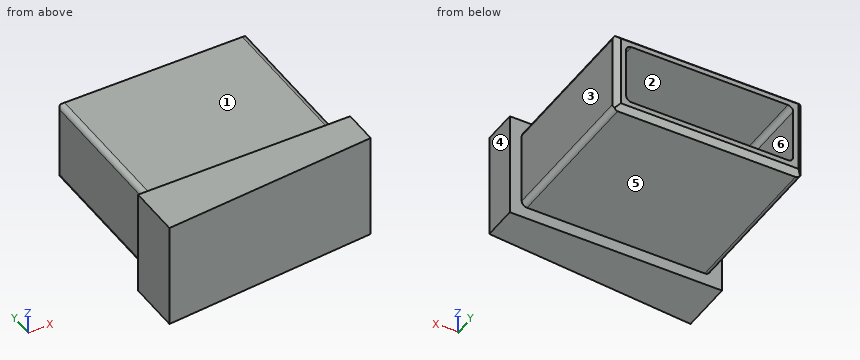
from build123d import *

# Parameters (mm, degrees)
SKETCH1_W           = 45.085
SKETCH1_H           = 38.1
BOSS_EXTRUDE1_DEPTH = 9.8425
SKETCH2_W           = 50.8
SKETCH2_H           = 25.4
BOSS_EXTRUDE2_DEPTH = 12.7635
CUT_EXTRUDE1_DEPTH  = 26.4
SKETCH4_W           = 40.005
SKETCH4_H           = 14.605
CUT_EXTRUDE2_DEPTH  = 38.1
CHAMFER1_SIZE       = 1.27
FILLET1_R           = 1.27


with BuildPart() as part:
    # Sketch1 → Boss-Extrude1 (new body, symmetric)
    with BuildSketch(Plane.XY):
        Rectangle(SKETCH1_W, SKETCH1_H)
    extrude(amount=BOSS_EXTRUDE1_DEPTH, both=True)

    # Sketch2 → Boss-Extrude2 (add)
    with BuildSketch(Plane.XZ.offset(19.05)):
        Rectangle(SKETCH2_W, SKETCH2_H)
    extrude(amount=BOSS_EXTRUDE2_DEPTH)

    # Sketch3 → Cut-Extrude1 (cut, through all)
    with BuildSketch(Plane.XY.offset(12.7)):
        Polygon((25.4, -31.8135), (25.4, -27.369075893), (-25.4, -31.8135), align=None)
    extrude(amount=-CUT_EXTRUDE1_DEPTH, mode=Mode.SUBTRACT)

    # Sketch4 → Cut-Extrude2 (cut)
    with BuildSketch(Plane(origin=(0, 19.05, 0), x_dir=(1, 0, 0), z_dir=(0, 1, 0))):
        Rectangle(SKETCH4_W, SKETCH4_H)
    extrude(amount=-CUT_EXTRUDE2_DEPTH, mode=Mode.SUBTRACT)

    # Chamfer1
    chamfer1_edges = [part.edges().sort_by_distance(p)[0] for p in [
        (0, 19.05, -9.8425),
        (-22.5425, 19.05, 0),
        (22.5425, 19.05, 0),
        (0, 19.05, 9.8425),
    ]]
    chamfer(chamfer1_edges, length=CHAMFER1_SIZE)

    # Fillet1
    fillet1_edges = [part.edges().sort_by_distance(p)[0] for p in [
        (20.0025, 0, -7.3025),
        (20.0025, 0, 7.3025),
        (-20.0025, 0, 7.3025),
        (-20.0025, 0, -7.3025),
        (22.5425, -0.635, 9.8425),
        (-22.5425, -0.635, -9.8425),
        (-22.5425, -0.635, 9.8425),
        (22.5425, -0.635, -9.8425),
    ]]
    fillet(fillet1_edges, radius=FILLET1_R)


solid = part.part
For this review, take the finished solid that the model builds, in its own axes (mm). Face numbers are marked on the shaded views. A direction names the side the tool comes from. Coordinates: 2 decimals unless noted, no trailing zeros. Order: outer loops, then holes, each group sorted by start corner. A loop starts at its lowest first (then second) coordinate and runs counter-clockwise, first axis right, second up. Notation, with made-up numbers: (77.25, -17) - (81.25, -17) arc R24 ccw to (81.25, 2) - close; hole circle Ø10 at (45.25, 12.25). An arc over 180 degrees is marked (long way). Use one line per item in the form item = value.
Q1. Consider section B-B (z = 4). Give the boundary of the cut face in (x, y).
Checked values:
outline = (-25.4, -31.81) - (25.4, -27.37) - (25.4, -19.05) - (22.54, -19.05) - (22.54, 17.78) - (21.27, 19.05) - (20, 19.05) - (20, -19.05) - (-20, -19.05) - (-20, 19.05) - (-21.27, 19.05) - (-22.54, 17.78) - (-22.54, -19.05) - (-25.4, -19.05) - close
Q2. For P1, Ø11, axis at x = 4, y = -0.5, coming from the -Z side; P2, Ø1.5, axis at y = 6.5, z = 7, coming from the -X side; P3, Ø1.5, axis at x = -11.5, z = 6, coming from the +Y side, all flat-tipped, find the tip position at first contact; note any pin that passes through.
Checked values:
P1 = -9.84
P2 = -22.54
P3 = -19.05
Q3. For probe 1 along Z at (x, y) = (9.5, 6.5); probe 2 along X at (y, z) = (-7.5, 1); probe 3 along X at (y, z) = (-1.5, 6.75), list the stretches that pass through material, from the lowest coordinate up. Write a range as from..to.
Checked values:
probe_1 = -9.84..-7.3, 7.3..9.84
probe_2 = -22.54..-20, 20..22.54
probe_3 = -22.54..-19.78, 19.78..22.54
Q4. Draft analysis for pull direction Z (two halves, no side actions). For the marked faces 4, 5 and 6, state which applies: +Z half, -Z half, draft (parallel to the pull), parting line (faces both ways), or undercut.
Checked values:
face_4 = draft
face_5 = -Z half
face_6 = undercut
Q5. For the marked faces 1, 2 and 3, list the 3-axis set-ups (+Z, -Z, +X, -X, +Y, -Y) from which the entire face can be reached by the end or side of a thin tool; tool diameter is ignored.
Checked values:
face_1 = +Z, +X, -X, +Y
face_2 = +Y
face_3 = +Z, -Z, +X, +Y
Q6. Consider section C-C (x = 2.5). Give the boundary of the cut face in (y, z).
Checked values:
outline = (-29.37, -12.7) - (-19.05, -12.7) - (-19.05, -9.84) - (17.78, -9.84) - (19.05, -8.57) - (19.05, -7.3) - (-19.05, -7.3) - (-19.05, 7.3) - (19.05, 7.3) - (19.05, 8.57) - (17.78, 9.84) - (-19.05, 9.84) - (-19.05, 12.7) - (-29.37, 12.7) - close
Q7. Consider section A-A (y = -10.5). Give the boundary of the cut face in (x, z), then the cut area to 3 significant figures.
Checked values:
outline = (-22.54, -8.57) arc R1.27 ccw to (-21.27, -9.84) - (21.27, -9.84) arc R1.27 ccw to (22.54, -8.57) - (22.54, 8.57) arc R1.27 ccw to (21.27, 9.84) - (-21.27, 9.84) arc R1.27 ccw to (-22.54, 8.57) - close; hole (-20, -6.03) arc R1.27 ccw to (-18.73, -7.3) - (18.73, -7.3) arc R1.27 ccw to (20, -6.03) - (20, 6.03) arc R1.27 ccw to (18.73, 7.3) - (-18.73, 7.3) arc R1.27 ccw to (-20, 6.03) - close
area = 303 mm2
